Source: three-view drawing plus pictorial views. Frame: mm from the lowest corner of the part. A direction names the side the tool comes from. Give positions to 0.01 mm unless a question says otherwise; leave off trailing zeros. Loops run counter-clockwise (first coordinate to the right, second up) from the corner with the lowest first, then second, coordinate; pieces in that order, holes last. Notation, with made-up numbers: M 61.5,34 L 112.5,34 A20 cw 112.5,46 Z; hole C 61,57 d1. An arc over 180 degrees is marked long. One line per item, written item: value. Start each with the question number.
(1) Section C-C on y = 7. Output: boundary loops of the cut face in (x, z) (1 decimal).
(2) Section D-D on x = 12. Output: boundary loops of the cut face in (y, z) (1 decimal).
(3) Section A-A on z = 18.5. Output: boundary loops of the cut face in (x, y).
(4) Ray query, line 1 along Z through (x, y) = (23, 16.5); line 2 along Y through (x, z) = (30.5, 10); line 3 along X through (y, z) = (15, 9). Return the intervals inside material, ascending. Write a range as from..to.
(5) Access query for the marked faces 1, 2 and 3. Directions: +Z, -Z, +X, -X, +Y, -Y. A direction counts if a zero-diameter tool reaches every point of the face in a straight line with its end or side. Return the directions, or none.
(6) Section B-B on x = 4. Output: boundary loops of the cut face in (y, z), plus the area to 3 significant figures.
(7) Pin query (flat end, axial travel): P1, Ø6, axis at x = 22, y = 6.5, coming from the +Z side; P2, Ø6.5, axis at x = 16.5, z = 39.5, coming from the +Y side; P3, Ø6, axis at x = 19, y = 32, coming from the +Z side; P4, Ø10, axis at y = 33.5, z = 28, coming from the +X side. Return the tip coordinate at first contact, or that it passes through.
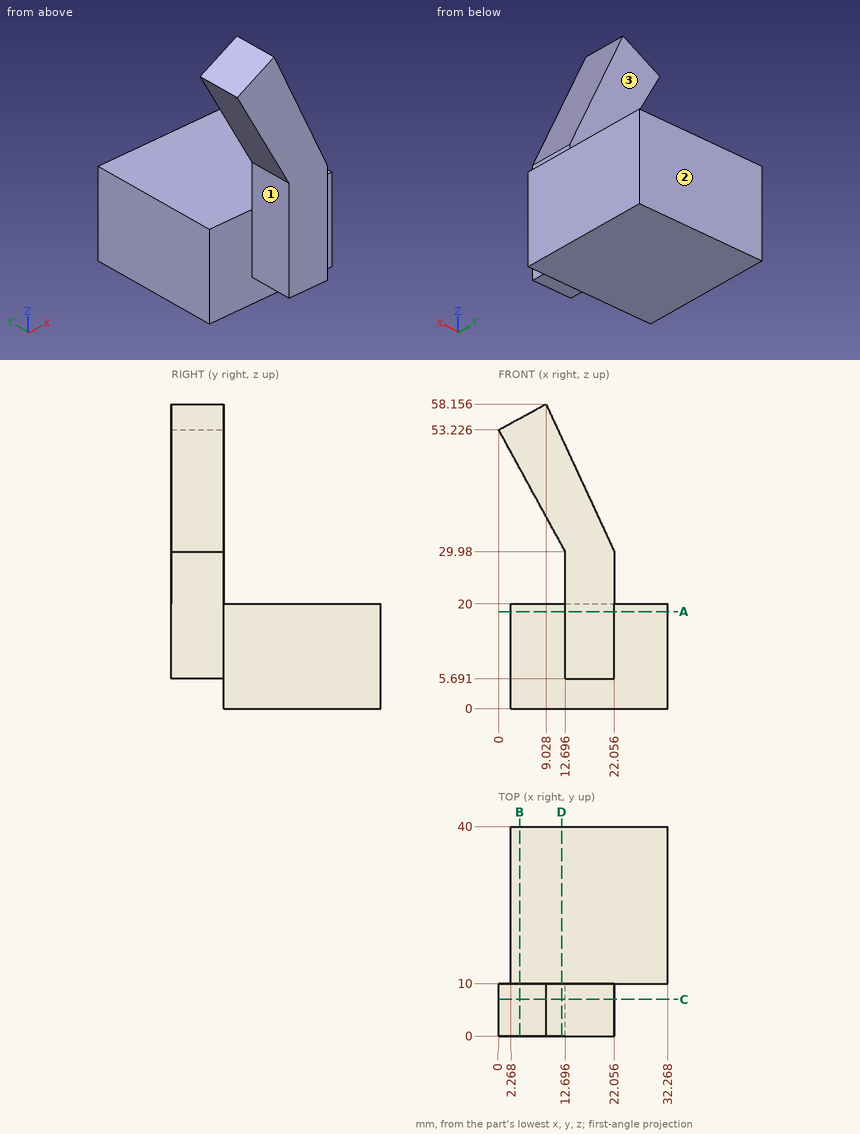
Output values:
1. outline: M 0,53.2 L 12.7,30 L 12.7,5.7 L 22.1,5.7 L 22.1,30 L 9,58.2 Z
2. outline: M 0,31.3 L 10,31.3 L 10,51.7 L 0,51.7 Z; M 10,0 L 40,0 L 40,20 L 10,20 Z
3. outline: M 2.27,10 L 12.7,10 L 12.7,0 L 22.06,0 L 22.06,10 L 32.27,10 L 32.27,40 L 2.27,40 Z
4. line 1: z = 0..20
4. line 2: y = 10..40
4. line 3: x = 2.27..32.27
5. face 1: -Z, -X, -Y
5. face 2: +Z, -Z, +X, -X, +Y
5. face 3: +Z, +X, -X, +Y
6. outline: M 0,45.9 L 10,45.9 L 10,55.41 L 0,55.41 Z; M 10,0 L 40,0 L 40,20 L 10,20 Z
6. area: 695 mm²
7. P1: stops at z = 36.59
7. P2: stops at y = 10
7. P3: stops at z = 20
7. P4: passes through
